Check sheet for the modelled part. Datum: model origin and axes. Units: mm. A direction names the side the tool comes from. Coordinates: 2 decimals unless noted, no trailing zeros. Loops run counter-clockwise (first coordinate to the right, second up) from the corner with the lowest first, then second, coordinate; pieces in that order, holes last.
```python
from build123d import *

# Parameters (mm, degrees)
CHAMFER_1_SIZE      = 2
CUT_EXTRUDE_START   = 11.75
SKETCH_3_W          = 22
SKETCH_3_H          = 5
CUT_EXTRUDE_1_DEPTH = 25
CUT_EXTRUDE_START_2 = 16
SKETCH_4_W          = 28
SKETCH_4_H          = 6
CUT_EXTRUDE_2_DEPTH = 11


with BuildPart() as part:
    # 草图2 → 旋转1 (revolve)
    with BuildSketch(Plane(origin=(0, 0, 0), x_dir=(1, 0, 0), z_dir=(0, 1, 0))):
        Polygon((0, 0), (0, 15), (40.5, 15), (40.5, 16), (96.5, 16), (96.5, 20), (136.5, 20), (136.5, 21.5), (139.5, 21.5), (139.5, 16), (152.1, 16), (152.1, 15), (184.1, 15), (184.1, 0), align=None)
    revolve(axis=Axis((184.1, 0, 0), (-1, 0, 0)))

    # 倒角1
    chamfer_1_edges = [part.edges().sort_by_distance(p)[0] for p in [
        (184.1, 0, 15),
        (0, 0, 15),
    ]]
    chamfer(chamfer_1_edges, length=CHAMFER_1_SIZE)

    # 草图3 → 切除-拉伸1 (cut)
    with BuildSketch(Plane(origin=(0, 0, 0), x_dir=(1, 0, 0), z_dir=(0, 1, 0)).offset(CUT_EXTRUDE_START)):
        with Locations((68.5, 2.5)):
            Rectangle(SKETCH_3_W, SKETCH_3_H)
        with Locations((68.5, -2.5)):
            Rectangle(SKETCH_3_W, SKETCH_3_H)
    extrude(amount=CUT_EXTRUDE_1_DEPTH, mode=Mode.SUBTRACT)

    # 草图4 → 切除-拉伸2 (cut)
    with BuildSketch(Plane(origin=(0, 0, 0), x_dir=(1, 0, 0), z_dir=(0, 1, 0)).offset(CUT_EXTRUDE_START_2)):
        with Locations((116.5, 3)):
            Rectangle(SKETCH_4_W, SKETCH_4_H)
        with Locations((116.5, -3)):
            Rectangle(SKETCH_4_W, SKETCH_4_H)
    extrude(amount=CUT_EXTRUDE_2_DEPTH, mode=Mode.SUBTRACT)


solid = part.part
```
1) Depth check by flat-ended pin: pin 1 (2.5 mm diameter, centred on x = 116.5, y = 17, fed in from -Z); pin 2 (1 mm diameter, centred on y = -12.5, z = 10.5, fed in from -X); pin 3 (1.5 mm diameter, centred on y = -15.5, z = 15, fed in from +X). Enter the tip coordinate at first touch or a pass-through.
Answer sheet:
pin 1: stops at z = -12.33
pin 2: stops at x = 40.5
pin 3: stops at x = 139.5
2) Section check A-A on y = 0. Enter the section's corners in (x, z), plus the area to 3 significant figures.
Answer sheet:
outline: (0, -13) - (2, -15) - (40.5, -15) - (40.5, -16) - (96.5, -16) - (96.5, -20) - (136.5, -20) - (136.5, -21.5) - (139.5, -21.5) - (139.5, -16) - (152.1, -16) - (152.1, -15) - (182.1, -15) - (184.1, -13) - (184.1, 13) - (182.1, 15) - (152.1, 15) - (152.1, 16) - (139.5, 16) - (139.5, 21.5) - (136.5, 21.5) - (136.5, 20) - (96.5, 20) - (96.5, 16) - (40.5, 16) - (40.5, 15) - (2, 15) - (0, 13) - close
area: 6,090 mm2
3) Section check B-B on x = 172. Enter the section's corners in (y, z), plus the area to 3 significant figures.
Answer sheet:
outline: circle Ø30 at (0, 0)
area: 707 mm2
4) Scan lines: line 1 (X direction, y = 17, z = 0); line 2 (X direction, y = -15.5, z = 0.5); line 3 (X direction, y = -12.5, z = -14). Record each from-to range of solid material in increasing order.
Answer sheet:
line 1: x = 96.5 to 102.5, 130.5 to 139.5
line 2: x = 40.5 to 152.1
line 3: x = 96.5 to 139.5
5) Set-up check for faces 1 (the cylindrical face through (116.78, -19.83, 2.6)), 2 (the cylindrical face through (145.89, 15.62, 3.47)), 3 (the flat face through (68, 13, 5)): record each of +Z, -Z, +X, -X, +Y, -Y from which the full face is reachable in a straight line by a thin tool's end or side.
Answer sheet:
face 1: -X
face 2: +X
face 3: +Y
6) Section check C-C on x = 108.5. Enter the section's corners in (y, z), plus the area to 3 significant figures.
Answer sheet:
outline: (16, -6) - (16, 6) - (19.08, 6) arc R20 ccw (long way) to (19.08, -6) - close
area: 1,210 mm2
7) Mould release check, pull along X, two halves, no side actions. Record for faces 4 (the flat face through (96.5, -13.43, -8.98)), 5 (the flat face through (139.5, -16, 3)), 6 (the cylindrical face through (21.52, -0.66, 14.985)), 7 (the flat face through (102.5, 18, 0)): +X half, -X half, draft (parallel to the pull), parting line (faces both ways), or undercut.
Answer sheet:
face 4: -X half
face 5: +X half
face 6: draft
face 7: undercut
